Input: dimensioned drawing with shaded views. Units: mm. Origin: part minimum x, y, z. A direction names the side the tool comes from. Give positions to 0.01 mm unless a question says otherwise; leave off trailing zeros. Loops run counter-clockwise (first coordinate to the right, second up) from the corner with the lowest first, then second, coordinate; pieces in that order, holes last.
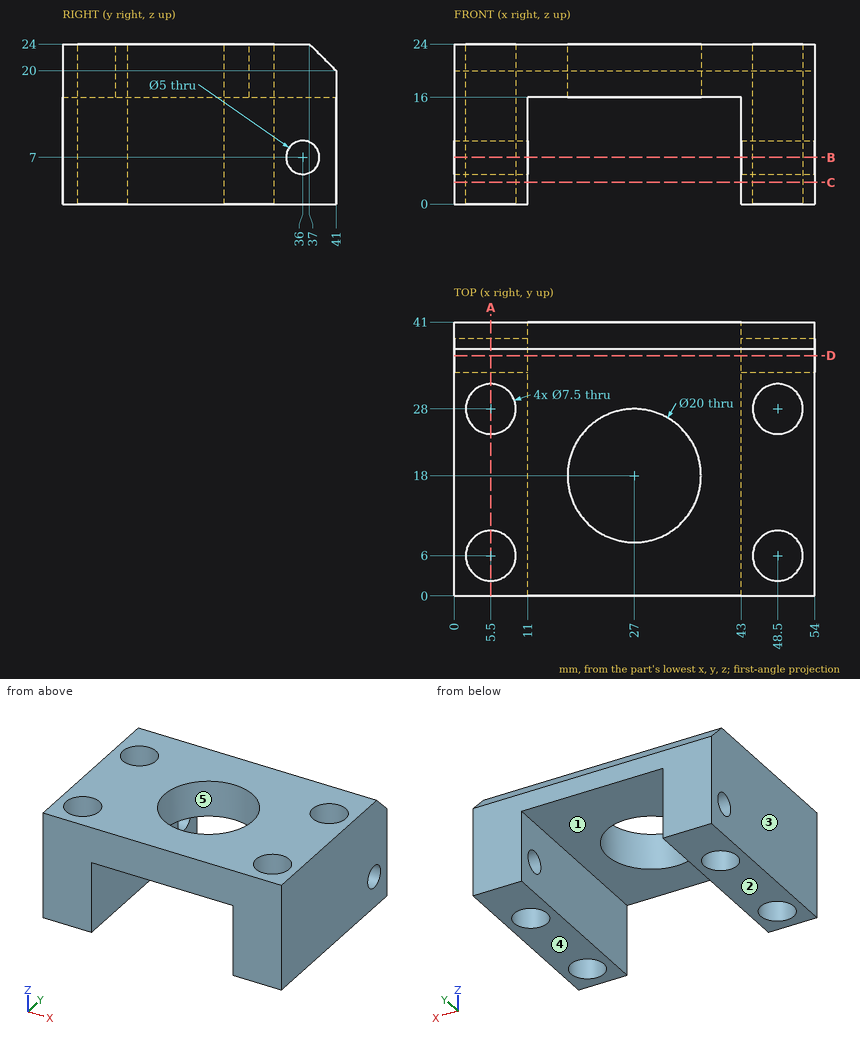
Item 1: Section query A-A on x = 5.5. Return loops of the section in (y, z), plus the area to 3 significant figures.
Values follow:
outline: (0, 0) - (2.25, 0) - (2.25, 24) - (0, 24) - close; (9.75, 0) - (24.25, 0) - (24.25, 24) - (9.75, 24) - close; (31.75, 0) - (41, 0) - (41, 20) - (37, 24) - (31.75, 24) - close; hole circle Ø5 at (36, 7)
area: 596 mm2
Item 2: Section query C-C on z = 3.25. Return loops of the section in (x, y), plus the area to 3 significant figures.
Values follow:
outline: (0, 0) - (11, 0) - (11, 41) - (0, 41) - close; (43, 0) - (54, 0) - (54, 41) - (43, 41) - close; hole circle Ø7.5 at (5.5, 6); hole circle Ø7.5 at (5.5, 28); hole circle Ø7.5 at (48.5, 6); hole circle Ø7.5 at (48.5, 28)
area: 725 mm2
Item 3: Draft query along X for the marked faces 3, 4 and 5. Return one class per face: +X half, -X half, draft (parallel to the pull), parting line (faces both ways), or undercut.
Values follow:
face 3: -X half
face 4: draft
face 5: undercut
Item 4: Section query D-D on y = 36. Return loops of the section in (x, z).
Values follow:
outline: (0, 0) - (11, 0) - (11, 4.5) - (0, 4.5) - close; (0, 9.5) - (11, 9.5) - (11, 16) - (43, 16) - (43, 9.5) - (54, 9.5) - (54, 24) - (0, 24) - close; (43, 0) - (54, 0) - (54, 4.5) - (43, 4.5) - close
Item 5: Pin query (flat end, axial travel): pin 1 (1.5 mm diameter, centred on x = 8, z = 21.5, fed in from +Y). Return the tip coordinate at first contact, or that it passes through.
Values follow:
pin 1: stops at y = 40.25
Item 6: Set-up query: the marked faces 1 and 2. Return all of +Z, -Z, +X, -X, +Y, -Y with unobstructed straight access to the full face (end or side cutting, diameter ignored); none if empty.
Values follow:
face 1: -Z, +Y, -Y
face 2: -Z, +X, -X, +Y, -Y
Item 7: Section query B-B on z = 7. Return loops of the section in (x, y).
Values follow:
outline: (0, 0) - (11, 0) - (11, 33.5) - (0, 33.5) - close; (0, 38.5) - (11, 38.5) - (11, 41) - (0, 41) - close; (43, 0) - (54, 0) - (54, 33.5) - (43, 33.5) - close; (43, 38.5) - (54, 38.5) - (54, 41) - (43, 41) - close; hole circle Ø7.5 at (5.5, 6); hole circle Ø7.5 at (5.5, 28); hole circle Ø7.5 at (48.5, 6); hole circle Ø7.5 at (48.5, 28)
Item 8: Ray query, probe 1 along X at (y, z) = (14, 8.75); probe 2 along Y at (x, z) = (5.5, 7.75); probe 3 along Z at (x, y) = (5, 36). Return the intervals inside material, ascending.
Values follow:
probe 1: x = 0 to 11, 43 to 54
probe 2: y = 0 to 2.25, 9.75 to 24.25, 31.75 to 33.62, 38.38 to 41
probe 3: z = 0 to 4.5, 9.5 to 24
